Here's the drawing with two shaded views (mm, measured from the low corner). I have some questions. A direction names the side the tool comes from. Coordinates: 2 decimals unless noted, no trailing zeros. Write each loop counter-clockwise with the first axis right and the second up, starting at its lowest first coordinate (ties: lowest second). Pieces come first, ordered by that corner, then holes. Notation, with made-up numbers: (-22.5, 33.25) -> (-10.5, 33.25) arc R11 ccw to (-10.5, 43.25) -> close; hole circle Ø4 at (71.25, 14). An arc over 180 degrees is marked (long way). Answer in a Markdown table with one row per item. Add a question column.
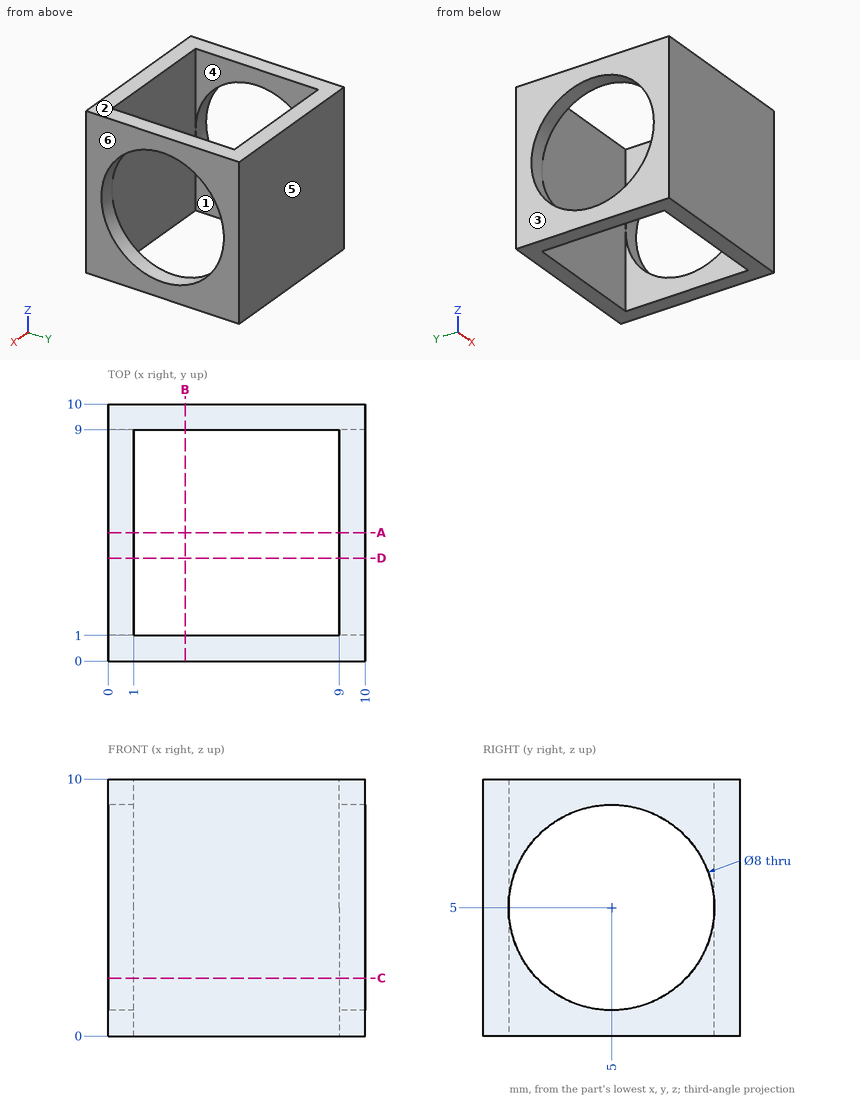
Q1. For the marked faces 1 and 2, which set-ups out of +Z, -Z, +X, -X, +Y, -Y let a thin tool reach every point of the face, with its end or its side?
Q2. Imagine slicing it at B-B on x = 3. Please give me the cut outline in (y, z), plus the area to 3 significant figures.
Q3. If we mould it in two halves opening along X, with no side actions, what happens to the marked faces 3, 4, 5 and 6? For each: pulls with the +X half, pulls with the -X half, needs draft (parallel to the pull), parting line crosses it, or undercut.
Q4. Imagine slicing it at D-D on y = 4. Please give me the cut outline in (x, z), plus the area to 3 significant figures.
Q5. Imagine slicing it at A-A on y = 5. Please give me the cut outline in (x, z), plus the area to 3 significant figures.
Q6. I need wall thicknesses on line 1 (Z direction, x = 9.5, y = 5). Which ranges of the line are inside material? Lowest first, please. Write a range as [from, to].
Q7. Imagine slicing it at C-C on z = 2.25. Please give me the cut outline in (x, y), plus the area to 3 significant figures.
Result sheet:
| question | item | result |
|---|---|---|
| 1 | face 1 | +Z, -Z |
| 1 | face 2 | +Z, +X, -X, +Y, -Y |
| 2 | outline | (0, 0) -> (1, 0) -> (1, 10) -> (0, 10) -> close; (9, 0) -> (10, 0) -> (10, 10) -> (9, 10) -> close |
| 2 | area | 20.0 mm^2 |
| 3 | face 3 | pulls with the -X half |
| 3 | face 4 | undercut |
| 3 | face 5 | needs draft |
| 3 | face 6 | pulls with the +X half |
| 4 | outline | (0, 0) -> (1, 0) -> (1, 1.13) -> (0, 1.13) -> close; (0, 8.87) -> (1, 8.87) -> (1, 10) -> (0, 10) -> close; (9, 0) -> (10, 0) -> (10, 1.13) -> (9, 1.13) -> close; (9, 8.87) -> (10, 8.87) -> (10, 10) -> (9, 10) -> close |
| 4 | area | 4.51 mm^2 |
| 5 | outline | (0, 0) -> (1, 0) -> (1, 1) -> (0, 1) -> close; (0, 9) -> (1, 9) -> (1, 10) -> (0, 10) -> close; (9, 0) -> (10, 0) -> (10, 1) -> (9, 1) -> close; (9, 9) -> (10, 9) -> (10, 10) -> (9, 10) -> close |
| 5 | area | 4.00 mm^2 |
| 6 | line 1 | z = [0, 1], [9, 10] |
| 7 | outline | (0, 0) -> (10, 0) -> (10, 2.1) -> (9, 2.1) -> (9, 1) -> (1, 1) -> (1, 2.1) -> (0, 2.1) -> close; (0, 7.9) -> (1, 7.9) -> (1, 9) -> (9, 9) -> (9, 7.9) -> (10, 7.9) -> (10, 10) -> (0, 10) -> close |
| 7 | area | 24.4 mm^2 |
